Answer from the drawing. Dimensions are ordinates in mm from the lowest x, y and z of the part. A direction names the side the tool comes from. Coordinates: 2 decimals unless noted, no trailing zeros. Write each loop counter-clockwise with the first axis right and the second up, starting at its lowest first coordinate (ties: lowest second). Pieces come first, ordered by that corner, then holes.
(1) Given P1, Ø6.5, axis at x = 37.5, y = 10, coming from the +Z side; P2, Ø7, axis at x = 37.5, z = 4.5, coming from the +Y side, each flat-ended and moving along its own axis, determine where each tip first touches the part or whether it passes through.
(2) The part is cut by section A-A on z = 12.5. Determine the outline of the cut face in (x, y), plus the area to 3 significant figures.
(3) The part is cut by section B-B on x = 37.5. Determine the outline of the cut face in (y, z).
(4) For a pull along Z with two mould halves and no side action, classify the marked faces 3, 4, 5 and 6 as +Z half, -Z half, draft (parallel to the pull), parting line (faces both ways), or undercut.
(5) Straight lines are drawn through the part: line 1 (Z direction, x = 12.5, y = 15.75); line 2 (Y direction, x = 37.5, z = 14.75); line 3 (Z direction, x = 14, y = 3). For each, find the intervals that lie inside material, in ascending order.
(6) The part is cut by section C-C on y = 3. Determine the outline of the cut face in (x, z).
(7) Which of the six approach directions +Z, -Z, +X, -X, +Y, -Y give full straight-line access (tool end or side, diameter ignored) to the marked faces 1 and 2?
(8) The part is cut by section D-D on y = 10. Determine the outline of the cut face in (x, z).
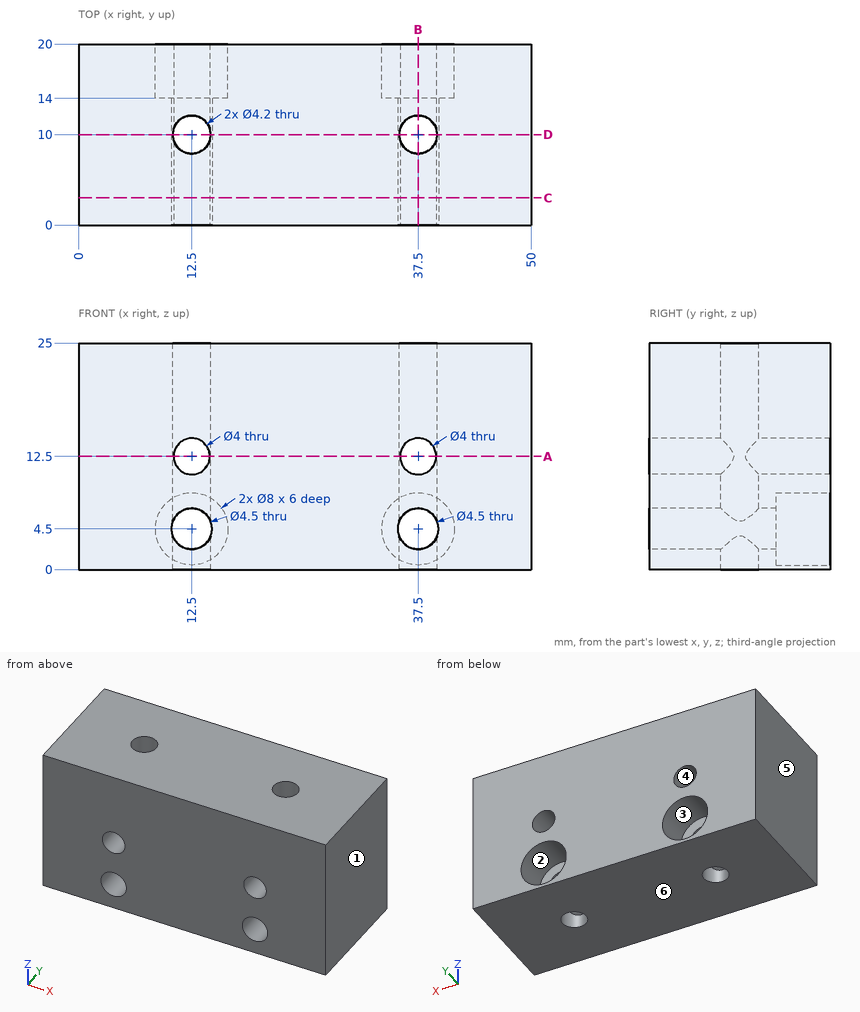
Model answer:
1. P1: stops at z = 25
1. P2: stops at y = 14
2. outline: (0, 0) - (10.5, 0) - (10.5, 9.36) arc R2.1 cw to (10.5, 10.64) - (10.5, 20) - (0, 20) - close; (14.5, 0) - (35.5, 0) - (35.5, 9.36) arc R2.1 cw to (35.5, 10.64) - (35.5, 20) - (14.5, 20) - (14.5, 10.64) arc R2.1 cw to (14.5, 9.36) - close; (39.5, 0) - (50, 0) - (50, 20) - (39.5, 20) - (39.5, 10.64) arc R2.1 cw to (39.5, 9.36) - close
2. area: 840 mm2
3. outline: (0, 0) - (7.9, 0) - (7.9, 2.25) - (0, 2.25) - close; (0, 6.75) - (7.9, 6.75) - (7.9, 10.5) - (0, 10.5) - close; (0, 14.5) - (7.9, 14.5) - (7.9, 25) - (0, 25) - close; (12.1, 0) - (20, 0) - (20, 0.5) - (14, 0.5) - (14, 2.25) - (12.1, 2.25) - close; (12.1, 6.75) - (14, 6.75) - (14, 8.5) - (20, 8.5) - (20, 10.5) - (12.1, 10.5) - close; (12.1, 14.5) - (20, 14.5) - (20, 25) - (12.1, 25) - close
4. face 3: undercut
4. face 4: undercut
4. face 5: draft
4. face 6: -Z half
5. line 1: z = 0 to 0.5, 8.5 to 10.5, 14.5 to 25
5. line 2: y = 0 to 7.9, 12.1 to 20
5. line 3: z = 0 to 2.82, 6.18 to 11.18, 13.82 to 25
6. outline: (0, 0) - (50, 0) - (50, 25) - (0, 25) - close; hole circle Ø4.5 at (12.5, 4.5); hole circle Ø4 at (12.5, 12.5); hole circle Ø4.5 at (37.5, 4.5); hole circle Ø4 at (37.5, 12.5)
7. face 1: +Z, -Z, +X, +Y, -Y
7. face 2: +Y
8. outline: (0, 0) - (10.4, 0) - (10.4, 3.69) arc R2.25 cw to (10.4, 5.31) - (10.4, 25) - (0, 25) - close; (14.6, 0) - (35.4, 0) - (35.4, 3.69) arc R2.25 cw to (35.4, 5.31) - (35.4, 25) - (14.6, 25) - (14.6, 5.31) arc R2.25 cw to (14.6, 3.69) - close; (39.6, 0) - (50, 0) - (50, 25) - (39.6, 25) - (39.6, 5.31) arc R2.25 cw to (39.6, 3.69) - close
